Here's how the part is built. I have some questions about the finished solid (model axes, mm). A direction names the side the tool comes from. Round coordinates to 2 decimals unless told otherwise and drop trailing zeros. Write each loop counter-clockwise with the first axis right and the second up, starting at its lowest first coordinate (ties: lowest second). Pieces come first, ordered by that corner, then holes. Notation, with made-up numbers: (22, -26.75) -> (46, -26.75) arc R5 cw to (46, -20.75) -> close; hole circle Ø5 at (31.25, 20.5). An arc over 180 degrees is marked (long way). Answer as CSV lines item,"result".
```python
from build123d import *

# Parameters (mm, degrees)
F2_R     = 1
F3_DEPTH = 8.79914
F4_R     = 2
F5_R     = 2


with BuildPart() as f1:
    # F0 (on Top) → F1 (revolve)
    with BuildSketch(Plane.XY):
        with BuildLine():
            Line((0, 3.79914), (0, 0))
            Line((0, 0), (15.723543, 0))
            Line((15.723543, 0), (15.723543, 8.79914))
            Line((15.723543, 8.79914), (11.849537, 8.79914))
            ThreePointArc((11.849537, 8.79914), (10.385071, 5.263606), (6.849537, 3.79914))
            Line((6.849537, 3.79914), (0, 3.79914))
        make_face()
    revolve(axis=Axis((0, 5, 0), (0, 1, 0)))

    # F2 (on face) → F3 (cut, through all)
    with BuildSketch(Plane(origin=(0, 8.79914, 0), x_dir=(-1, 0, 0), z_dir=(0, 1, 0))):
        with BuildLine():
            ThreePointArc((0, 2.785922), (0.363636, 2.762088), (0.72105, 2.690994))
            Line((0.72105, 2.690994), (1.772791, 6.616145))
            ThreePointArc((1.772791, 6.616145), (0.894044, 6.790939), (0, 6.849537))
            Line((0, 6.849537), (0, 2.785922))
        make_face()
        with BuildLine():
            ThreePointArc((-3.424769, 5.931873), (-4.169734, 5.434103), (-4.843354, 4.843354))
            Line((-4.843354, 4.843354), (-1.969944, 1.969944))
            ThreePointArc((-1.969944, 1.969944), (-1.695962, 2.21022), (-1.392961, 2.412679))
            Line((-1.392961, 2.412679), (-3.424769, 5.931873))
        make_face()
        with BuildLine():
            ThreePointArc((-6.616145, 1.772791), (-6.790939, 0.894044), (-6.849537, 0))
            Line((-6.849537, 0), (-2.785922, 0))
            ThreePointArc((-2.785922, 0), (-2.762088, 0.363636), (-2.690994, 0.72105))
            Line((-2.690994, 0.72105), (-6.616145, 1.772791))
        make_face()
        with BuildLine():
            ThreePointArc((-5.931873, -3.424769), (-5.434103, -4.169734), (-4.843354, -4.843354))
            Line((-4.843354, -4.843354), (-1.969944, -1.969944))
            ThreePointArc((-1.969944, -1.969944), (-2.21022, -1.695962), (-2.412679, -1.392961))
            Line((-2.412679, -1.392961), (-5.931873, -3.424769))
        make_face()
        with BuildLine():
            ThreePointArc((-1.772791, -6.616145), (-0.894044, -6.790939), (0, -6.849537))
            Line((0, -6.849537), (0, -2.785922))
            ThreePointArc((0, -2.785922), (-0.363636, -2.762088), (-0.72105, -2.690994))
            Line((-0.72105, -2.690994), (-1.772791, -6.616145))
        make_face()
        with BuildLine():
            ThreePointArc((3.424769, -5.931873), (4.169734, -5.434103), (4.843354, -4.843354))
            Line((4.843354, -4.843354), (1.969944, -1.969944))
            ThreePointArc((1.969944, -1.969944), (1.695962, -2.21022), (1.392961, -2.412679))
            Line((1.392961, -2.412679), (3.424769, -5.931873))
        make_face()
        with BuildLine():
            ThreePointArc((6.616145, -1.772791), (6.790939, -0.894044), (6.849537, 0))
            Line((6.849537, 0), (2.785922, 0))
            ThreePointArc((2.785922, 0), (2.762088, -0.363636), (2.690994, -0.72105))
            Line((2.690994, -0.72105), (6.616145, -1.772791))
        make_face()
        with BuildLine():
            ThreePointArc((5.931873, 3.424769), (5.434103, 4.169734), (4.843354, 4.843354))
            Line((4.843354, 4.843354), (1.969944, 1.969944))
            ThreePointArc((1.969944, 1.969944), (2.21022, 1.695962), (2.412679, 1.392961))
            Line((2.412679, 1.392961), (5.931873, 3.424769))
        make_face()
        Circle(F2_R)
    extrude(amount=-F3_DEPTH, mode=Mode.SUBTRACT)

    # F4
    f4_edges = [f1.edges().sort_by_distance(p)[0] for p in [
        (-15.723543, 8.79914, 0),
    ]]
    fillet(f4_edges, radius=F4_R)

    # F5
    f5_edges = [f1.edges().sort_by_distance(p)[0] for p in [
        (-15.723543, 0, 0),
    ]]
    fillet(f5_edges, radius=F5_R)


solid = f1.part
```
1. On a 3-axis mill with a long thin cutter (end or side, diameter ignored), from which of +Z, -Z, +X, -X, +Y, -Y can I reach the whole of each face in a straight line? I mean faces 3 (the face through (-12, 8.799, 0)), 4 (the face through (1.4, 3.799, -0.1)), 5 (the face through (5.44, 1.93, -4.16)). Say none if no direction works.
Numbers:
face 3,"+Z, -Z, +X, -X, +Y"
face 4,"+Y"
face 5,"+Y, -Y"
2. Suppose I cut it at C-C on y = 5.75. Please give me the cut outline in (x, z).
Numbers:
outline,"circle Ø31.45 at (0, 0); hole circle Ø21.62 at (0, 0)"
3. Suppose I cut it at A-A on y = 3. Count the separate pieces of the cut face and the enclosed holes in it, and give its area (3 significant figures).
Numbers:
separate pieces,"1"
enclosed holes,"9"
area,"733 mm^2"
4. If I drill on line 1 (X direction, y = 2.5, z = 0.5); line 2 (Z direction, x = 6.5, y = 8.25); line 3 (Z direction, x = -2, y = 7.25), over which ranges is the centre line in solid material (lowest first)?
Numbers:
line 1,"x = -15.72 to -0.87, 0.87 to 2.74, 6.83 to 15.72"
line 2,"z = -13.63 to -9.87, 9.87 to 13.63"
line 3,"z = -15.54 to -11.43, 11.43 to 15.54"
5. For pin 1 Ø7 at (x, z) = (1.5, -1.5) entering from +Y; pin 2 Ø4 at (x, y) = (2.5, 1) entering from +Z; pin 3 Ø1.9 at (x, y) = (4, 2.5) entering from +Z; pin 4 Ø1.8 at (x, z) = (0, 0) entering from -Y, each with a flat end and sliding along its axis, tell me the tip position at first contact or that it passes through.
Numbers:
pin 1,"stops at y = 3.8"
pin 2,"stops at z = 15.71"
pin 3,"stops at z = 15.42"
pin 4,"passes through"
6. If we mould it in two halves opening along Z, with no side actions, what happens to faces 1 (the face through (0, 2, 5)), 2 (the face through (0.2, 0, 2.9))? For each: released by +Z, released by -Z, zero draft, split by the parting line, or undercut.
Numbers:
face 1,"undercut"
face 2,"zero draft"
